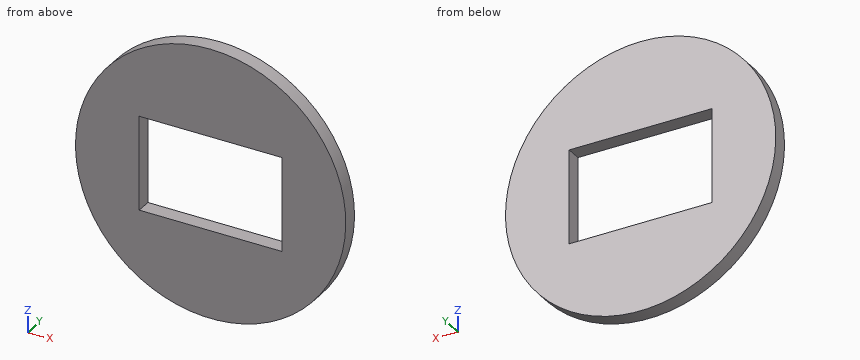
```python
from build123d import *

# Parameters (mm, degrees)
SKETCH1_R           = 88.9
BOSS_EXTRUDE1_DEPTH = 10
SKETCH2_W           = 94
SKETCH2_H           = 62
CUT_EXTRUDE1_DEPTH  = 30


with BuildPart() as part:
    # Sketch1 → Boss-Extrude1 (new body)
    with BuildSketch(Plane(origin=(0, 0, 0), x_dir=(1, 0, 0), z_dir=(0, 1, 0))):
        with Locations(Location((0, 0, 0), (0, 0, 270))):
            Circle(SKETCH1_R)
    extrude(amount=BOSS_EXTRUDE1_DEPTH)

    # Sketch2 → Cut-Extrude1 (cut)
    with BuildSketch(Plane.XZ.offset(10)):
        Rectangle(SKETCH2_W, SKETCH2_H)
    extrude(amount=-CUT_EXTRUDE1_DEPTH, mode=Mode.SUBTRACT)


solid = part.part
```
For this review, take the finished solid that the model builds, in its own axes (mm). Coordinates: 2 decimals unless noted, no trailing zeros. Write each loop counter-clockwise with the first axis right and the second up, starting at its lowest first coordinate (ties: lowest second). Pieces come first, ordered by that corner, then holes.
(1) Add section B-B on x = 0. Give the boundary of the cut face in (y, z), then the cut area to 3 significant figures.
(2) Add section A-A on z = 0. Give the boundary of the cut face in (x, y).
(3) Add section C-C on y = 3.5. Give the boundary of the cut face in (x, z).
(4) Add section D-D on z = -57. Give the boundary of the cut face in (x, y).
(5) For pin 1 Ø3 at (y, z) = (2, -63.5) entering from +X; pin 2 Ø3 at (x, y) = (-4, 5.5) entering from +Z; pin 3 Ø3 at (x, y) = (-15, 3) entering from +Z, all flat-tipped, find the tip position at first contact; note any pin that passes through.
(6) Wall thickness on probe 1 along X at (y, z) = (3, 0.5); probe 2 along X at (y, z) = (3.5, -14); probe 3 along Z at (x, y) = (11, 2): over which ranges is each line inside the solid? List them lowest first.
Answer sheet:
1. outline: (0, -88.9) - (10, -88.9) - (10, -31) - (0, -31) - close; (0, 31) - (10, 31) - (10, 88.9) - (0, 88.9) - close
1. area: 1,160 mm2
2. outline: (-88.9, 0) - (-47, 0) - (-47, 10) - (-88.9, 10) - close; (47, 0) - (88.9, 0) - (88.9, 10) - (47, 10) - close
3. outline: circle Ø177.8 at (0, 0); hole (-47, -31) - (47, -31) - (47, 31) - (-47, 31) - close
4. outline: (-68.22, 0) - (68.22, 0) - (68.22, 10) - (-68.22, 10) - close
5. pin 1: stops at x = 63.71
5. pin 2: stops at z = 88.86
5. pin 3: stops at z = 87.87
6. probe 1: x = -88.9 to -47, 47 to 88.9
6. probe 2: x = -87.79 to -47, 47 to 87.79
6. probe 3: z = -88.22 to -31, 31 to 88.22
